```python
from build123d import *

# Parameters (mm, degrees)
SKETCH1_W           = 196
SKETCH1_H           = 6
BOSS_EXTRUDE1_DEPTH = 50
SKETCH2_W           = 6
SKETCH2_H           = 6
BOSS_EXTRUDE2_DEPTH = 6
SKETCH3_W           = 6
SKETCH3_H           = 6
CUT_EXTRUDE1_DEPTH  = 6
SKETCH5_W           = 6
SKETCH5_H           = 6
CUT_EXTRUDE2_DEPTH  = 6


with BuildPart() as part:
    # Sketch1 → Boss-Extrude1 (new body)
    with BuildSketch(Plane.XY):
        with Locations((0, 3)):
            Rectangle(SKETCH1_W, SKETCH1_H)
    extrude(amount=BOSS_EXTRUDE1_DEPTH)

    # Sketch2 → Boss-Extrude2 (add)
    with BuildSketch(Plane(origin=(0, 0, 0), x_dir=(-1, 0, 0), z_dir=(0, 0, -1))):
        with Locations((-89, 3)):
            Rectangle(SKETCH2_W, SKETCH2_H)
        with Locations((-38, 3)):
            Rectangle(SKETCH2_W, SKETCH2_H)
        with Locations((38, 3)):
            Rectangle(SKETCH2_W, SKETCH2_H)
        with Locations((89, 3)):
            Rectangle(SKETCH2_W, SKETCH2_H)
    extrude(amount=BOSS_EXTRUDE2_DEPTH)

    # Sketch3 → Cut-Extrude1 (cut)
    with BuildSketch(Plane(origin=(0, 6, 0), x_dir=(1, 0, 0), z_dir=(0, 1, 0))):
        with Locations((75, -47)):
            Rectangle(SKETCH3_W, SKETCH3_H)
        with Locations((24, -47)):
            Rectangle(SKETCH3_W, SKETCH3_H)
        with Locations((-24, -47)):
            Rectangle(SKETCH3_W, SKETCH3_H)
        with Locations((-75, -47)):
            Rectangle(SKETCH3_W, SKETCH3_H)
    extrude(amount=-CUT_EXTRUDE1_DEPTH, mode=Mode.SUBTRACT)

    # Sketch5 → Cut-Extrude2 (cut)
    with BuildSketch(Plane.XZ):
        with Locations((-19.5, 30.5)):
            Rectangle(SKETCH5_W, SKETCH5_H)
        with Locations((19.5, 30.5)):
            Rectangle(SKETCH5_W, SKETCH5_H)
    extrude(amount=-CUT_EXTRUDE2_DEPTH, mode=Mode.SUBTRACT)


solid = part.part
```
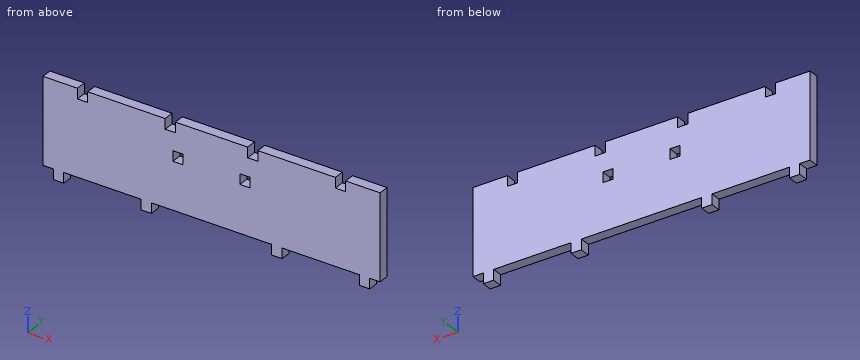
Geometry check sheet. Reference: the model listing, model coordinates, mm. Give positions to 0.01 mm unless a question says otherwise; leave off trailing zeros. Order: outer loops, then holes, each group sorted by start corner. A loop starts at its lowest first (then second) coordinate and runs counter-clockwise, first axis right, second up. Notation, with made-up numbers: (12.25, -2.5) -> (39.25, -2.5) arc R36 cw to (39.25, 34.5) -> close; hole circle Ø3 at (53, -22). An arc over 180 degrees is marked (long way). Write each question's results on one line, items separated by ' | '. Start each with the question number.
(1) Sectioned sample at C-C (y = 4.95). Give the number of separate pieces and of enclosed holes in the cut face, plus the area to 3 significant figures.
(2) Gauge pin test, flat ends, axial feed: P1, Ø1.8, axis at y = 1.5, z = -2.5, coming from the -X side; P2, Ø1.8, axis at x = -95, y = 3.5, coming from the -Z side. Record the tip position at first contact, or that the pin passes through.
(3) Sectioned sample at B-B (z = 46.5). Enter the section's corners in (x, y), plus the area to 3 significant figures.
(4) Scan line: line 1 (Z direction, x = -80, y = 1.2). Record every from-to range of solid material in increasing order.
(5) Sectioned sample at D-D (x = 49.5). Enter the section's corners in (y, z), plus the area to 3 significant figures.
(6) Sectioned sample at A-A (z = 30.5). Enter the section's corners in (x, y).
Answer below:
1) separate pieces: 1 | enclosed holes: 2 | area: 9,730 mm2
2) P1: x = -92 | P2: z = 0
3) outline: (-98, 0) -> (-78, 0) -> (-78, 6) -> (-98, 6) -> close; (-72, 0) -> (-27, 0) -> (-27, 6) -> (-72, 6) -> close; (-21, 0) -> (21, 0) -> (21, 6) -> (-21, 6) -> close; (27, 0) -> (72, 0) -> (72, 6) -> (27, 6) -> close; (78, 0) -> (98, 0) -> (98, 6) -> (78, 6) -> close | area: 1,030 mm2
4) line 1: 0 to 50
5) outline: (0, 0) -> (6, 0) -> (6, 50) -> (0, 50) -> close | area: 300 mm2
6) outline: (-98, 0) -> (-22.5, 0) -> (-22.5, 6) -> (-98, 6) -> close; (-16.5, 0) -> (16.5, 0) -> (16.5, 6) -> (-16.5, 6) -> close; (22.5, 0) -> (98, 0) -> (98, 6) -> (22.5, 6) -> close
